CAD build for the part. Positions are in the model's coordinates, mm. Face numbers are marked on the shaded views. A direction names the side the tool comes from. Coordinates: 2 decimals unless noted, no trailing zeros. Order: outer loops, then holes, each group sorted by start corner. A loop starts at its lowest first (then second) coordinate and runs counter-clockwise, first axis right, second up. Notation, with made-up numbers: M -29,-31 L -16,-31 A7 ccw -16,-22 Z; hole C 54.5,30.25 d2. An arc over 180 degrees is marked long. Write item = value, one per line. Start each with the question number.
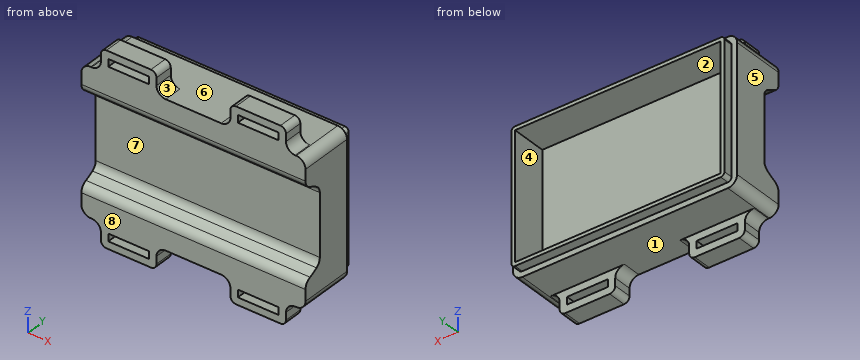
```python
from build123d import *

# Parameters (mm, degrees)
CROQUIS2_W                   = 121
CROQUIS2_H                   = 78
CROQUIS2_W_2                 = 111
CROQUIS2_H_2                 = 68
SALIENTE_EXTRUIR2_DEPTH      = 19
CROQUIS4_W                   = 121
CROQUIS4_H                   = 78
SALIENTE_EXTRUIR3_DEPTH      = 5
SALIENTE_EXTRUIR4_DEPTH      = 60.5
SALIENTE_EXTRUIR4_DEPTH_BACK = 60.5
REDONDEO2_R                  = 5
CROQUIS7_W                   = 30
CROQUIS7_H                   = 12
CROQUIS7_W_2                 = 22
CROQUIS7_H_2                 = 4
SALIENTE_EXTRUIR5_DEPTH      = 10
REDONDEO5_R                  = 3
REDONDEO8_R                  = 5
REDONDEO6_R                  = 5
CROQUIS8_OUTSIDE_W           = 155.374
CROQUIS8_OUTSIDE_H           = 136.374
CORTAR_EXTRUIR1_DEPTH        = 5


with BuildPart() as part:
    # Croquis2 → Saliente-Extruir2 (new body)
    with BuildSketch(Plane(origin=(0, 0, 0), x_dir=(1, 0, 0), z_dir=(0, 1, 0))):
        Rectangle(CROQUIS2_W, CROQUIS2_H)
        Rectangle(CROQUIS2_W_2, CROQUIS2_H_2, mode=Mode.SUBTRACT)
    extrude(amount=-SALIENTE_EXTRUIR2_DEPTH)

    # Croquis4 → Saliente-Extruir3 (add)
    with BuildSketch(Plane.XZ.offset(19)):
        Rectangle(CROQUIS4_W, CROQUIS4_H)
    extrude(amount=SALIENTE_EXTRUIR3_DEPTH)

    # Croquis6 → Saliente-Extruir4 (add, two sides: drawn at the far end of the back side and taken through both)
    with BuildSketch(Plane(origin=(0, 0, 0), x_dir=(0, 0, -1), z_dir=(1, 0, 0)).offset(-SALIENTE_EXTRUIR4_DEPTH_BACK)):
        with BuildLine():
            Line((-39, -24), (-19.209372712, -24))
            ThreePointArc((-19.209372712, -24), (-22.306932281, -28.712804945), (-24.269322199, -34))
            Line((-24.269322199, -34), (-39, -34))
            Line((-39, -34), (-39, -24))
        make_face()
        with BuildLine():
            Line((39, -24), (39, -34))
            Line((39, -34), (24.269322199, -34))
            ThreePointArc((24.269322199, -34), (22.306932281, -28.712804945), (19.209372712, -24))
            Line((19.209372712, -24), (39, -24))
        make_face()
    extrude(amount=SALIENTE_EXTRUIR4_DEPTH + SALIENTE_EXTRUIR4_DEPTH_BACK)

    # Redondeo2
    redondeo2_edges = [part.edges().sort_by_distance(p)[0] for p in [
        (0, -34, 24.269322199),
        (0, -24, 19.209372712),
        (0, -34, -24.269322199),
        (0, -24, -19.209372712),
    ]]
    fillet(redondeo2_edges, radius=REDONDEO2_R)

    # Croquis7 → Saliente-Extruir5 (add)
    # profile 1 of 4: a face of its own
    with BuildSketch(Plane.XZ.offset(24)):
        with Locations((-34.974984355, 45)):
            Rectangle(CROQUIS7_W, CROQUIS7_H)
        with Locations((-34.974984355, 45)):
            Rectangle(CROQUIS7_W_2, CROQUIS7_H_2, mode=Mode.SUBTRACT)
    # profile 2 of 4: a face of its own
    with BuildSketch(Plane.XZ.offset(24)):
        with Locations((-34.974984355, -45)):
            Rectangle(CROQUIS7_W, CROQUIS7_H)
        with Locations((-34.974984355, -45)):
            Rectangle(CROQUIS7_W_2, CROQUIS7_H_2, mode=Mode.SUBTRACT)
    # profile 3 of 4: a face of its own
    with BuildSketch(Plane.XZ.offset(24)):
        with Locations((34.974984355, -45)):
            Rectangle(CROQUIS7_W, CROQUIS7_H)
        with Locations((34.974984355, -45)):
            Rectangle(CROQUIS7_W_2, CROQUIS7_H_2, mode=Mode.SUBTRACT)
    # profile 4 of 4: a face of its own
    with BuildSketch(Plane.XZ.offset(24)):
        with Locations((34.974984355, 45)):
            Rectangle(CROQUIS7_W, CROQUIS7_H)
        with Locations((34.974984355, 45)):
            Rectangle(CROQUIS7_W_2, CROQUIS7_H_2, mode=Mode.SUBTRACT)
    extrude(amount=SALIENTE_EXTRUIR5_DEPTH)

    # Redondeo5
    redondeo5_edges = [part.edges().sort_by_distance(p)[0] for p in [
        (-49.974984355, -29, 51),
        (-19.974984355, -29, 51),
        (-49.974984355, -29, -51),
        (-19.974984355, -29, -51),
        (19.974984355, -29, -51),
        (49.974984355, -29, -51),
        (49.974984355, -29, 51),
        (19.974984355, -29, 51),
    ]]
    fillet(redondeo5_edges, radius=REDONDEO5_R)

    # Redondeo8
    redondeo8_edges = [part.edges().sort_by_distance(p)[0] for p in [
        (60.5, -17, 39),
        (-60.5, -17, 39),
        (-60.5, -17, -39),
        (60.5, -17, -39),
    ]]
    fillet(redondeo8_edges, radius=REDONDEO8_R)

    # Redondeo6
    redondeo6_edges = [part.edges().sort_by_distance(p)[0] for p in [
        (-49.974984355, -29, 39),
        (-19.974984355, -29, 39),
        (-49.974984355, -29, -39),
        (-19.974984355, -29, -39),
        (49.974984355, -29, -39),
        (19.974984355, -29, -39),
        (49.974984355, -29, 39),
        (19.974984355, -29, 39),
    ]]
    fillet(redondeo6_edges, radius=REDONDEO6_R)

    # Croquis8 outside → Cortar-Extruir1 (cut)
    with BuildSketch(Plane(origin=(0, 0, 0), x_dir=(1, 0, 0), z_dir=(0, 1, 0))):
        Rectangle(CROQUIS8_OUTSIDE_W, CROQUIS8_OUTSIDE_H)
        with BuildLine():
            Line((55.5, 36), (-55.5, 36))
            ThreePointArc((-55.5, 36), (-56.914213562, 35.414213562), (-57.5, 34))
            Line((-57.5, 34), (-57.5, -34))
            ThreePointArc((-57.5, -34), (-56.914213562, -35.414213562), (-55.5, -36))
            Line((-55.5, -36), (55.5, -36))
            ThreePointArc((55.5, -36), (56.914213562, -35.414213562), (57.5, -34))
            Line((57.5, -34), (57.5, 34))
            ThreePointArc((57.5, 34), (56.914213562, 35.414213562), (55.5, 36))
        make_face(mode=Mode.SUBTRACT)
    extrude(amount=-CORTAR_EXTRUIR1_DEPTH, mode=Mode.SUBTRACT)


solid = part.part
```
1. Slice it at D-D (x = 0). Write the cut outline in (y, z), plus the area to 3 significant figures.
2. Mould opens along Z. For the marked faces 1, 2 and 3 say: released by +Z, released by -Z, zero draft, split by the parting line, or undercut.
3. Probe L1, parallel to X at y = -18.5, z = -26.5; L2, parallel to Z at x = 24, y = -10; L3, parallel to X at y = -4.5, z = 24.5. List the from-to ranges inside material, lowest first.
4. Flat gauge pins, fed straight in: pin 1 (4.5 mm diameter, centred on y = -31, z = 46.5, fed in from +X) (3 decimals); pin 2 (4 mm diameter, centred on x = -39, y = -6.5, fed in from -Z); pin 3 (4 mm diameter, centred on x = -10.5, z = -2, fed in from +Y). Where does each tip first touch, or does it go through?
5. Slice it at B-B (y = -17). Write the cut outline in (x, z).
6. 3-axis set-ups, long thin cutter, end or side, ignore diameter. For the marked faces 4, 5, 6, 7 and 8: which of +Z, -Z, +X, -X, +Y, -Y reach the whole face in a straight line?
7. Slice it at C-C (z = 2). Write the cut outline in (x, y), plus the area to 3 significant figures.
8. Slice it at A-A (x = -33). Give the number of separate pieces and of enclosed holes in the cut face, plus the area to 3 significant figures.
Calculated:
q1.outline = M -34,-39 L -5,-39 L -5,-36 L 0,-36 L 0,-34 L -19,-34 L -19,34 L 0,34 L 0,36 L -5,36 L -5,39 L -34,39 L -34,27.91 A5 ccw -30.83,23.26 A25 cw -26.25,20.88 A5 cw -24,16.7 L -24,-16.7 A5 cw -26.25,-20.88 A25 cw -30.83,-23.26 A5 ccw -34,-27.91 Z
q1.area = 883 mm²
q2.face_1 = released by -Z
q2.face_2 = undercut
q2.face_3 = released by +Z
q3.L1 = -60.5 to -55.5, 55.5 to 60.5
q3.L2 = -39 to -34, 34 to 39
q3.L3 = -57.5 to -55.5, 55.5 to 57.5
q4.pin_1 = 49.975
q4.pin_2 = -39
q4.pin_3 = -19
q5.outline = M -60.5,-34 A5 ccw -55.5,-39 L 55.5,-39 A5 ccw 60.5,-34 L 60.5,34 A5 ccw 55.5,39 L -55.5,39 A5 ccw -60.5,34 Z; hole M -55.5,-34 L 55.5,-34 L 55.5,34 L -55.5,34 Z
q6.face_4 = +Y
q6.face_5 = +Z, -Z, -X, +Y, -Y
q6.face_6 = +Z, +Y
q6.face_7 = +X, -X, -Y
q6.face_8 = +Z, -Z, +X, -X, -Y
q7.outline = M -60.5,-24 L 60.5,-24 L 60.5,-5 L 57.5,-5 L 57.5,0 L 55.5,0 L 55.5,-19 L -55.5,-19 L -55.5,0 L -57.5,0 L -57.5,-5 L -60.5,-5 Z
q7.area = 765 mm²
q8.separate_pieces = 3
q8.enclosed_holes = 0
q8.area = 1,040 mm²
